Solid Edge part; units mm, degrees
sketch "Sketch1" plane through (0, 0, 0) normal (0, 0, 1) x (1, 0, 0)
  circle A0 centre (0, 0) radius 50
extrude "Protrusion1" add sketch "Sketch1" along normal blind 450
sketch "Sketch2" plane through (0, 0, 0) normal (0, -1, 0) x (1, 0, 0)
  line L0 (25.5502, -35.238) -> (25.5502, 5.2165)
  line L1 (25.5502, 5.2165) -> (-44.4999, 5.2165)
  line L2 (-44.4999, 5.2165) -> (-44.4999, -35.238)
  line L3 (-44.4999, -35.238) -> (25.5502, -35.238)
extrude "Cutout1" cut sketch "Sketch2" along normal up to next
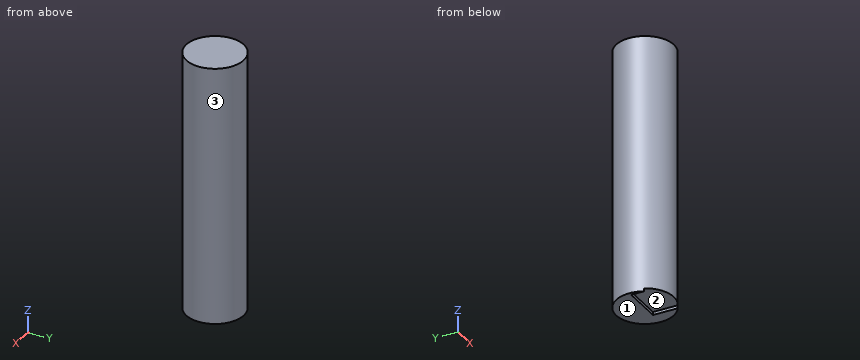
The model under review builds one solid part; all positions refer to its coordinate system, in mm. Face numbers are marked on the shaded views. Give positions to 0.01 mm unless a question says otherwise; leave off trailing zeros. Write each loop counter-clockwise with the first axis right and the second up, starting at its lowest first coordinate (ties: lowest second). Pieces come first, ordered by that corner, then holes.
(1) To check wall thickness, follow L1, parallel to X at y = -3, z = 39.5; L2, parallel to Z at x = -21, y = -5; L3, parallel to Y at x = -2.5, z = 422. State the ranges of each line that lie inside material, in increasing order.
(2) Consider section C-C, the plane y = -12.5. Give the boundary of the cut face in (x, z), and give its area (3 significant figures).
(3) For P1, Ø5.5, axis at x = -24, z = 2, coming from the -Y side; P2, Ø2.5, axis at y = -14, z = 3.5, coming from the -X side; P3, Ø1.5, axis at y = -28.5, z = 235, coming from the +X side, all flat-tipped, find the tip position at first contact; note any pin that passes through.
(4) Consider section B-B, the plane z = 286.5. Give the boundary of the cut face in (x, y), and give its area (3 significant figures).
(5) The part is to be moulded in two halves that separate along X. For the marked faces 1, 2 and 3, say which applies: released by +X, released by -X, zero draft, split by the parting line, or undercut.
(6) Consider section A-A, the plane x = 7.5. Give the boundary of the cut face in (y, z), and give its area (3 significant figures).
(7) Consider section D-D, the plane x = -36. Give the boundary of the cut face in (y, z), and give its area (3 significant figures).
Returned:
1. L1: x = -49.91 to 49.91
1. L2: z = 5.22 to 450
1. L3: y = -49.94 to 49.94
2. outline: (-48.41, 0) - (-44.5, 0) - (-44.5, 5.22) - (25.55, 5.22) - (25.55, 0) - (48.41, 0) - (48.41, 450) - (-48.41, 450) - close
2. area: 43,200 mm2
3. P1: stops at y = 0
3. P2: stops at x = -48.35
3. P3: stops at x = 41.59
4. outline: circle Ø100 at (0, 0)
4. area: 7,850 mm2
5. face 1: zero draft
5. face 2: undercut
5. face 3: split by the parting line
6. outline: (-49.43, 5.22) - (0, 5.22) - (0, 0) - (49.43, 0) - (49.43, 450) - (-49.43, 450) - close
6. area: 44,200 mm2
7. outline: (-34.7, 5.22) - (0, 5.22) - (0, 0) - (34.7, 0) - (34.7, 450) - (-34.7, 450) - close
7. area: 31,000 mm2
